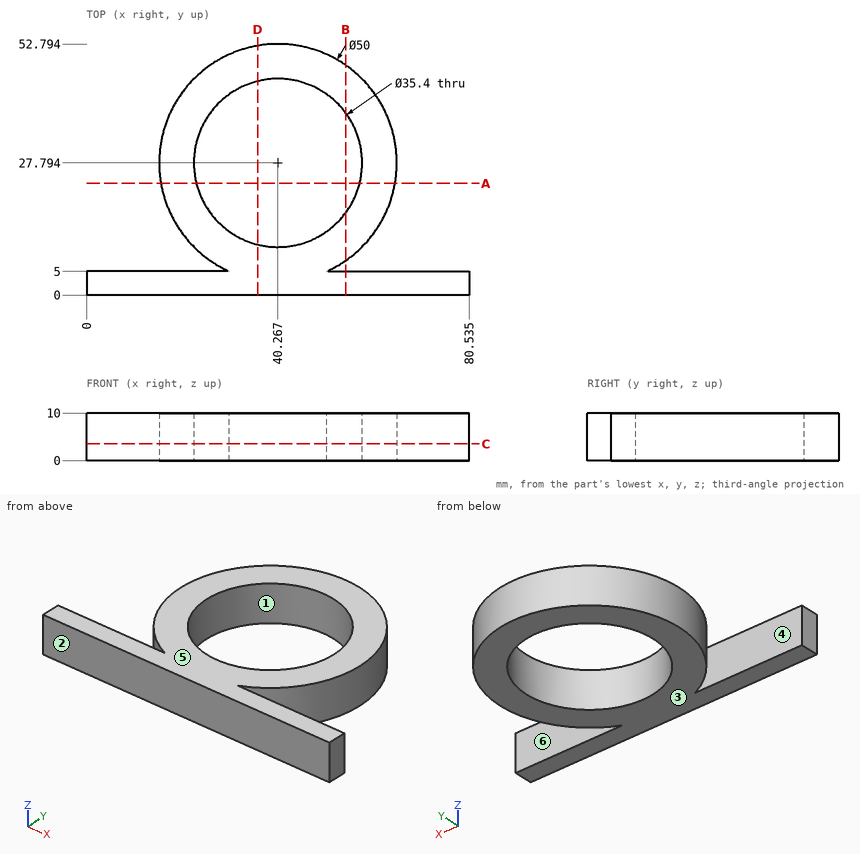
The drawing under review shows one solid part. Ordinate dimensions are in mm from its lowest x, y, z. A direction names the side the tool comes from. Coordinates: 2 decimals unless noted, no trailing zeros. Write each loop counter-clockwise with the first axis right and the second up, starting at its lowest first coordinate (ties: lowest second). Pieces come first, ordered by that corner, then holes. Notation, with made-up numbers: (70, 45.25) - (80, 45.25) arc R17 ccw to (80, 71.25) - close; hole circle Ø10 at (87, -6.5). An arc over 180 degrees is marked (long way). Use one line per item in the form item = value.
Q1. Machinability: for the marked faces 4, 5 and 6, which of the approach directions +Z, -Z, +X, -X, +Y, -Y give a long, thin tool a straight path to every point of the face, cutting with its end or side? Answer none if there is none.
Taken from the geometry:
face_4 = +Z, -Z, -X
face_5 = +Z, +X, -X, +Y, -Y
face_6 = +Z, -Z, +X
Q2. The part is to be moulded in two halves that separate along Y. For the marked faces 1, 2 and 3, say which applies: +Y half, -Y half, draft (parallel to the pull), parting line (faces both ways), or undercut.
Taken from the geometry:
face_1 = undercut
face_2 = -Y half
face_3 = draft
Q3. Consider section C-C (z = 3.5). Write out the cut boundary in (x, y) (1 decimal), plus the area to 3 significant figures.
Taken from the geometry:
outline = (0, 0) - (80.5, 0) - (80.5, 5) - (50.5, 5) arc R25 ccw (long way) to (30, 5) - (0, 5) - close; hole circle Ø35.4 at (40.3, 27.8)
area = 1,350 mm^2
Q4. Consider section B-B (x = 54.5). Write out the cut boundary in (y, z).
Taken from the geometry:
outline = (0, 0) - (5, 0) - (5, 10) - (0, 10) - close; (7.24, 0) - (17.27, 0) - (17.27, 10) - (7.24, 10) - close; (38.32, 0) - (48.35, 0) - (48.35, 10) - (38.32, 10) - close
Q5. Insertion check: pin 1 Ø3 at (y, z) = (30, 3) entering from +X; pin 2 Ø3 at (x, z) = (60, 5.5) entering from +Y; pin 3 Ø5 at (x, z) = (20.5, 5) entering from +Y. Each pin has a flat end and moves straight along its axis. Give the tip position at first contact, or say it passes through.
Taken from the geometry:
pin_1 = 65.26
pin_2 = 44.9
pin_3 = 45.87
Q6. Consider section A-A (y = 23.5). Write out the cut boundary in (x, z).
Taken from the geometry:
outline = (15.64, 0) - (23.1, 0) - (23.1, 10) - (15.64, 10) - close; (57.44, 0) - (64.9, 0) - (64.9, 10) - (57.44, 10) - close
Q7. For probe 1 along Y at (x, z) = (8, 5.5); probe 2 along Y at (x, z) = (40, 1); probe 3 along Y at (x, z) = (36.5, 4.5), list the stretches that pass through material, from the lowest coordinate up.
Taken from the geometry:
probe_1 = 0 to 5
probe_2 = 0 to 10.1, 45.49 to 52.79
probe_3 = 0 to 10.5, 45.09 to 52.51
Q8. Consider section D-D (x = 36). Write out the cut boundary in (y, z), plus the area to 3 significant figures.
Taken from the geometry:
outline = (0, 0) - (10.62, 0) - (10.62, 10) - (0, 10) - close; (44.97, 0) - (52.43, 0) - (52.43, 10) - (44.97, 10) - close
area = 181 mm^2
